```python
from build123d import *

# Parameters (mm, degrees)
BOSS_EXTRUDE1_DEPTH = 25
SKETCH2_W           = 57.7
SKETCH2_H           = 16.5
CUT_EXTRUDE1_DEPTH  = 51.363081717
SKETCH3_W           = 30
SKETCH3_H           = 20
CUT_EXTRUDE2_DEPTH  = 7.5
CUT_EXTRUDE3_REACH  = 57.579
SKETCH4_R           = 2
SKETCH5_R           = 2
CUT_EXTRUDE4_DEPTH  = 1.5
SKETCH6_W           = 6
SKETCH6_H           = 8
BOSS_EXTRUDE2_DEPTH = 2
BOSS_EXTRUDE4_DEPTH = 6
SKETCH9_W           = 32
SKETCH9_H           = 22
CUT_EXTRUDE5_DEPTH  = 2
FILLET1_R           = 1
SKETCH10_R          = 1
BOSS_EXTRUDE5_DEPTH = 1.5
FILLET3_R           = 1
SKETCH7_W           = 4
SKETCH7_H           = 18.7
BOSS_EXTRUDE6_DEPTH = 2
FILLET4_R           = 1
SKETCH11_W          = 4.5
SKETCH11_H          = 2
BOSS_EXTRUDE7_DEPTH = 2.5
SKETCH12_W          = 0.5
SKETCH12_H          = 4.68
BOSS_EXTRUDE8_DEPTH = 2.5
CUT_EXTRUDE6_REACH  = 80.825


with BuildPart() as part:
    # Sketch1 → Boss-Extrude1 (new body)
    with BuildSketch(Plane.XY):
        Polygon((0, 0), (30, 0), (30, -7.7), (-32.7, -7.7), (-32.7, -26.2), (35, -26.2), (35, 9), (0, 9), align=None)
    extrude(amount=BOSS_EXTRUDE1_DEPTH)

    # Sketch2 → Cut-Extrude1 (cut, through all)
    with BuildSketch(Plane.XY.offset(25)):
        with Locations((1.15, -17.95)):
            Rectangle(SKETCH2_W, SKETCH2_H)
    extrude(amount=-CUT_EXTRUDE1_DEPTH, mode=Mode.SUBTRACT)

    # Sketch3 → Cut-Extrude2 (cut)
    with BuildSketch(Plane(origin=(0, 9, 0), x_dir=(1, 0, 0), z_dir=(0, 1, 0))):
        with Locations((17.5, -12.5)):
            Rectangle(SKETCH3_W, SKETCH3_H)
    extrude(amount=-CUT_EXTRUDE2_DEPTH, mode=Mode.SUBTRACT)

    # Cut-Extrude3: up to this face of the body (flat: up to its plane)
    cut_extrude3_end = Plane(part.part.faces().sort_by_distance((17.5, 1.5, 12.5))[0])
    # Sketch4 → Cut-Extrude3 (cut, up to the picked face)
    with BuildSketch(Plane.XZ.offset(26.2), mode=Mode.PRIVATE) as cut_extrude3_sk1:
        with Locations(Location((30.5, 12.5, 0), (0, 0, 255.522487814))):
            Circle(SKETCH4_R)
    cut_extrude3_tool1 = split(extrude(cut_extrude3_sk1.sketch, amount=-CUT_EXTRUDE3_REACH, mode=Mode.PRIVATE), bisect_by=cut_extrude3_end, keep=Keep.BOTH, mode=Mode.PRIVATE)
    add(cut_extrude3_tool1.solids().sort_by(Axis((30.5, -26.2, 12.5), (0, 1, 0)))[0], mode=Mode.SUBTRACT)

    # Sketch5 → Cut-Extrude4 (cut)
    with BuildSketch(Plane(origin=(0, 1.5, 0), x_dir=(1, 0, 0), z_dir=(0, 1, 0))):
        with Locations(Location((5, -15, 0), (0, 0, 180))):
            Circle(SKETCH5_R)
    extrude(amount=-CUT_EXTRUDE4_DEPTH, mode=Mode.SUBTRACT)

    # Sketch6 → Boss-Extrude2 (add)
    with BuildSketch(Plane.XZ.offset(26.2)):
        with Locations((32, 21)):
            Rectangle(SKETCH6_W, SKETCH6_H)
        with Locations((32, 4)):
            Rectangle(SKETCH6_W, SKETCH6_H)
        with Locations((-29.7, 12.5)):
            Rectangle(SKETCH6_W, SKETCH6_H)
    extrude(amount=BOSS_EXTRUDE2_DEPTH)

    # Sketch8 → Boss-Extrude4 (add)
    with BuildSketch(Plane(origin=(35, 0, 0), x_dir=(0, 0, -1), z_dir=(1, 0, 0))):
        Polygon((-25, -28.2), (0, -31.86), (0, -28.2), align=None)
    extrude(amount=-BOSS_EXTRUDE4_DEPTH)

    # Sketch9 → Cut-Extrude5 (cut)
    with BuildSketch(Plane(origin=(0, 9, 0), x_dir=(1, 0, 0), z_dir=(0, 1, 0))):
        with Locations((17.5, -12.5)):
            Rectangle(SKETCH9_W, SKETCH9_H)
    extrude(amount=-CUT_EXTRUDE5_DEPTH, mode=Mode.SUBTRACT)

    # Fillet1
    fillet1_edges = [part.edges().sort_by_distance(p)[0] for p in [
        (33.5, 8, 1.5),
        (33.5, 8, 23.5),
        (1.5, 8, 23.5),
        (1.5, 8, 1.5),
        (2.5, 4.25, 22.5),
        (2.5, 4.25, 2.5),
        (32.5, 4.25, 2.5),
        (32.5, 4.25, 22.5),
    ]]
    fillet(fillet1_edges, radius=FILLET1_R)

    # Sketch10 → Boss-Extrude5 (add)
    with BuildSketch(Plane(origin=(-27.7, 0, 0), x_dir=(0, 0, -1), z_dir=(1, 0, 0))):
        with Locations(Location((-14, -12.05, 0), (0, 0, 180))):
            Circle(SKETCH10_R)
        with Locations(Location((-11, -12.05, 0), (0, 0, 180))):
            Circle(SKETCH10_R)
    extrude(amount=BOSS_EXTRUDE5_DEPTH)

    # Fillet3
    fillet3_edges = [part.edges().sort_by_distance(p)[0] for p in [
        (-26.2, -12.05, 13),
        (-26.2, -12.05, 10),
    ]]
    fillet(fillet3_edges, radius=FILLET3_R)

    # Sketch7 → Boss-Extrude6 (add)
    with BuildSketch(Plane.XY):
        with Locations((2, -0.35)):
            Rectangle(SKETCH7_W, SKETCH7_H)
    extrude(amount=-BOSS_EXTRUDE6_DEPTH)

    # Fillet4
    fillet4_edges = [part.edges().sort_by_distance(p)[0] for p in [
        (4, -8.7, 0),
        (4, 4.5, 0),
    ]]
    fillet(fillet4_edges, radius=FILLET4_R)
    fillet4_2_edges = [part.edges().sort_by_distance(p)[0] for p in [
        (-29.7, -28.2, 16.5),
        (-26.7, -28.2, 12.5),
        (-29.7, -28.2, 8.5),
        (-32.7, -28.2, 12.5),
        (32, -31.86, 0),
        (32, -28.2, 25),
        (29, -30.03, 12.5),
        (35, -30.03, 12.5),
        (-30.2, -26.2, 0),
        (-30.2, -26.2, 25),
        (29, -29.03, 0),
        (29, -27.2, 25),
        (-26.7, -27.2, 8.5),
        (-26.7, -27.2, 16.5),
        (-32.7, -27.2, 8.5),
        (-32.7, -27.2, 16.5),
        (-32.7, -26.2, 4.25),
        (-32.7, -26.2, 20.75),
        (-32.7, -16.95, 0),
        (-32.7, -16.95, 25),
        (-32.7, -7.7, 12.5),
        (4, -0.35, -2),
        (2, -9.7, -2),
        (20, 9, 0),
        (2, 9, -2),
        (0, -0.35, -2),
        (0, 9, 11.5),
        (0, 4.5, 25),
        (17.5, 9, 25),
        (35, 9, 12.5),
        (35, -9.6, 25),
        (35, -11.43, 0),
        (4.292893219, 9, -0.292893219),
    ]]
    fillet(fillet4_2_edges, radius=FILLET4_R - 0.0001)  # a hair under: the kernel refuses the full size

    # Sketch11 → Boss-Extrude7 (add)
    with BuildSketch(Plane(origin=(0, 1.5, 0), x_dir=(1, 0, 0), z_dir=(0, 1, 0))):
        with Locations((4.75, -18.34)):
            Rectangle(SKETCH11_W, SKETCH11_H)
        with Locations((4.75, -11.66)):
            Rectangle(SKETCH11_W, SKETCH11_H)
    extrude(amount=BOSS_EXTRUDE7_DEPTH)

    # Sketch12 → Boss-Extrude8 (add)
    with BuildSketch(Plane(origin=(0, 1.5, 0), x_dir=(1, 0, 0), z_dir=(0, 1, 0))):
        with Locations((2.75, -15)):
            Rectangle(SKETCH12_W, SKETCH12_H)
    extrude(amount=BOSS_EXTRUDE8_DEPTH)

    # Cut-Extrude6: up to this face of the body (flat: up to its plane)
    cut_extrude6_end = Plane(part.part.faces().sort_by_distance((32.5, 4.25, 12.5))[0])
    # Sketch13 → Cut-Extrude6 (cut, up to the picked face)
    with BuildSketch(Plane(origin=(35, 0, 0), x_dir=(0, 0, -1), z_dir=(1, 0, 0)), mode=Mode.PRIVATE) as cut_extrude6_sk1:
        with BuildLine():
            Line((-9.5, 9), (-9.5, 4.5))
            ThreePointArc((-9.5, 4.5), (-7, 2), (-4.5, 4.5))
            Line((-4.5, 4.5), (-4.5, 9))
            Line((-4.5, 9), (-9.5, 9))
        make_face()
    cut_extrude6_tool1 = split(extrude(cut_extrude6_sk1.sketch, amount=-CUT_EXTRUDE6_REACH, mode=Mode.PRIVATE), bisect_by=cut_extrude6_end, keep=Keep.BOTH, mode=Mode.PRIVATE)
    add(cut_extrude6_tool1.solids().sort_by(Axis((35, 5.744167, 7), (-1, 0, 0)))[0], mode=Mode.SUBTRACT)


solid = part.part
```
Could you check a few things on this model? Use its own coordinates, in mm. A direction names the side the tool comes from. Round coordinates to 2 decimals unless told otherwise and drop trailing zeros. Loops run counter-clockwise (first coordinate to the right, second up) from the corner with the lowest first, then second, coordinate; pieces in that order, holes last. Notation, with made-up numbers: (22, -14) - (37, -14) arc R22 cw to (37, 5) - close; hole circle Ø7 at (63.5, 35). An arc over 180 degrees is marked (long way). Answer in a Markdown table with one row per item. Add a question column.
(1) For faces 1 (the face through (7, 3, 12)), 2 (the face through (32, -27, 17)), 3 (the face through (35, -11, 13)), which set-ups out of +Z, -Z, +X, -X, +Y, -Y let a thin tool reach every point of the face, with its end or its side?
(2) If we mould it in two halves opening along Z, with no side actions, what happens to faces 4 (the face through (5, 3, 17.34)), 5 (the face through (32.028, -29.985, 12.806)), 6 (the face through (-22, -9, 0))? For each: pulls with the +Z half, pulls with the -Z half, needs draft (parallel to the pull), parting line crosses it, or undercut.
(3) If we section it at C-C (y = -20): Please give me the cut outline in (x, z), plus the area to 3 significant figures.
(4) If we section it at B-B (x = 23.5): Please give me the cut outline in (y, z).
(5) I'm going to push flat-ended pins straight in: pin 1 (5 mm diameter, centred on x = -22, z = 6, fed in from +Y); pin 2 (1.5 mm diameter, centred on x = -16.5, y = -7, fed in from -Z); pin 3 (4 mm diameter, centred on x = 16, z = 15.5, fed in from +Y). Where does each tip first touch, or does it pass through?
(6) I need wall thicknesses on line 1 along X through (y, z) = (-12, 12.5); line 2 along Y through (x, z) = (9.5, 17.5); line 3 along Z through (x, y) = (5, 1.1). Which ranges of each line are inside material? Lowest first, please.
(7) If we section it at D-D (x = -19): Please give me the cut outline in (y, z), plus the area to 3 significant figures.
(8) If we section it at A-A (y = -12.05): Please give me the cut outline in (x, z), plus the area to 3 significant figures.
Model answer:
| question | item | result |
|---|---|---|
| 1 | face 1 | +Y |
| 1 | face 2 | +X, -X |
| 1 | face 3 | +Z, -Z, +X, +Y, -Y |
| 2 | face 4 | undercut |
| 2 | face 5 | pulls with the +Z half |
| 2 | face 6 | pulls with the -Z half |
| 3 | outline | (-32.7, 1) arc R1 ccw to (-31.7, 0) - (-27.7, 0) - (-27.7, 25) - (-31.7, 25) arc R1 ccw to (-32.7, 24) - close; (30, 0) - (34, 0) arc R1 ccw to (35, 1) - (35, 24) arc R1 ccw to (34, 25) - (30, 25) - (30, 14.44) arc R2 cw (long way) to (30, 10.56) - close |
| 3 | area | 241 mm² |
| 4 | outline | (-9.7, 0) - (-7.7, 0) - (-7.7, 25) - (-9.7, 25) - close; (0, 0) - (8, 0) arc R1 ccw to (9, 1) - (9, 1.5) - (7, 1.5) - (7, 2.5) - (1.5, 2.5) - (1.5, 22.5) - (7, 22.5) - (7, 23.5) - (9, 23.5) - (9, 24) arc R1 ccw to (8, 25) - (0, 25) - close |
| 5 | pin 1 | stops at y = -7.7 |
| 5 | pin 2 | stops at z = 0 |
| 5 | pin 3 | stops at y = 1.5 |
| 6 | line 1 | x = -32.7 to -27.7, 32.5 to 35 |
| 6 | line 2 | y = -9.7 to -7.7, 0 to 1.5 |
| 6 | line 3 | z = 0 to 13, 17 to 25 |
| 7 | outline | (-9.7, 0) - (-7.7, 0) - (-7.7, 25) - (-9.7, 25) - close |
| 7 | area | 50.0 mm² |
| 8 | outline | (-32.7, 1) arc R1 ccw to (-31.7, 0) - (-27.7, 0) - (-27.7, 10) - (-27.2, 10) arc R1 ccw to (-27.2, 12) - (-27.7, 12) - (-27.7, 13) - (-27.2, 13) arc R1 ccw to (-27.2, 15) - (-27.7, 15) - (-27.7, 25) - (-31.7, 25) arc R1 ccw to (-32.7, 24) - close; (30, 0) - (34, 0) arc R1 ccw to (35, 1) - (35, 24) arc R1 ccw to (34, 25) - (30, 25) - (30, 14.44) arc R2 cw (long way) to (30, 10.56) - close |
| 8 | area | 246 mm² |
